Build history of the part. All positions in model axes, mm. Face numbers are marked on the shaded views. A direction names the side the tool comes from. Coordinates: 2 decimals unless noted, no trailing zeros. Write each loop counter-clockwise with the first axis right and the second up, starting at its lowest first coordinate (ties: lowest second). Pieces come first, ordered by that corner, then holes.
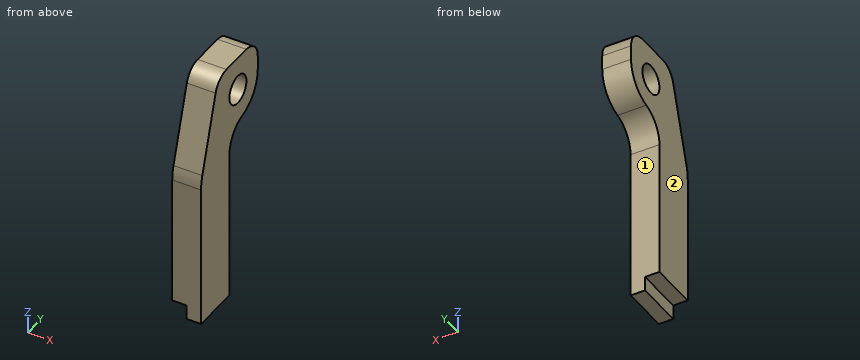
```python
from build123d import *

# Parameters (mm, degrees)
TAB_EXTRUDE_DEPTH       = 5
SKETCH2_R               = 1.5
SCREWHOLE_EXTRUDE_DEPTH = 3
STRUCTURAL_FILLETS_R    = 5


with BuildPart() as part:
    # Sketch1 → Tab extrude (new body)
    with BuildSketch(Plane(origin=(0, 116.5, 0), x_dir=(1, 0, 0), z_dir=(0, 1, 0))):
        Polygon((-4, 23.815), (-2.5, 23.815), (-2.5, 25.315), (-1, 25.315), (-1, 9.63955532), (-4, 9.63955532), align=None)
    extrude(amount=-TAB_EXTRUDE_DEPTH)

    # Sketch2 → Screwhole extrude (add)
    with BuildSketch(Plane.ZY.offset(1)):
        with BuildLine():
            Line((-9.63955532, 111.5), (-1.230909725, 114.067641584))
            ThreePointArc((-1.230909725, 114.067641584), (-0.207489417, 114.790530608), (0.185, 115.980450657))
            Line((0.185, 115.980450657), (0.185, 119.5))
            ThreePointArc((0.185, 119.5), (-0.400786438, 120.914213562), (-1.815, 121.5))
            Line((-1.815, 121.5), (-3.315, 121.5))
            ThreePointArc((-3.315, 121.5), (-5.485607855, 120.745625892), (-6.720529788, 118.807692308))
            ThreePointArc((-6.720529788, 118.807692308), (-7.779034301, 117.146606378), (-9.63955532, 116.5))
            Line((-9.63955532, 116.5), (-9.63955532, 111.5))
        make_face()
        with Locations((-3.315, 118)):
            Circle(SKETCH2_R, mode=Mode.SUBTRACT)
    extrude(amount=SCREWHOLE_EXTRUDE_DEPTH)

    # Structural fillets
    structural_fillets_edges = [part.edges().sort_by_distance(p)[0] for p in [
        (-2.5, 111.5, -9.63955532),
    ]]
    fillet(structural_fillets_edges, radius=STRUCTURAL_FILLETS_R)


solid = part.part
```
1. Flat gauge pins, fed straight in: pin 1 (1.6 mm diameter, centred on y = 114, z = -25, fed in from -X); pin 2 (1.5 mm diameter, centred on x = -3, z = -15, fed in from +Y). Where does each tip first touch, or does it go through?
Computed values:
pin 1: stops at x = -2.5
pin 2: stops at y = 116.5
2. Saw through at B-B on y = 118. List the corners of the cut face in (x, z) (3 decimals).
Computed values:
outline: (-4, -7.041) - (-1, -7.041) - (-1, -4.815) - (-4, -4.815) - close; (-4, -1.815) - (-1, -1.815) - (-1, 0.185) - (-4, 0.185) - close
3. Saw through at A-A on x = -1.8. List the corners of the cut face in (y, z) (3 decimals), plus the area to 3 significant figures.
Computed values:
outline: (111.5, -25.315) - (116.5, -25.315) - (116.5, -9.64) arc R3 cw to (118.808, -6.721) arc R3.5 ccw to (121.5, -3.315) - (121.5, -1.815) arc R2 ccw to (119.5, 0.185) - (115.98, 0.185) arc R2 ccw to (114.068, -1.231) - (111.718, -8.926) arc R5 ccw to (111.5, -10.386) - close; hole circle Ø3 at (118, -3.315)
area: 138 mm2
4. Saw through at D-D on x = -2.9. List the corners of the cut face in (y, z) (3 decimals).
Computed values:
outline: (111.5, -23.815) - (116.5, -23.815) - (116.5, -9.64) arc R3 cw to (118.808, -6.721) arc R3.5 ccw to (121.5, -3.315) - (121.5, -1.815) arc R2 ccw to (119.5, 0.185) - (115.98, 0.185) arc R2 ccw to (114.068, -1.231) - (111.718, -8.926) arc R5 ccw to (111.5, -10.386) - close; hole circle Ø3 at (118, -3.315)
5. 3-axis set-ups, long thin cutter, end or side, ignore diameter. For the marked faces 1 and 2: which of +Z, -Z, +X, -X, +Y, -Y reach the whole face in a straight line?
Computed values:
face 1: -Z, +X, -X, +Y
face 2: +Z, -Z, -X, +Y, -Y
6. Saw through at C-C on z = -20.25. List the corners of the cut face in (x, y), plus the area to 3 significant figures.
Computed values:
outline: (-4, 111.5) - (-1, 111.5) - (-1, 116.5) - (-4, 116.5) - close
area: 15.0 mm2
7. Probe line 1 along Y through (x, z) = (-2.85, -21.25); line 2 along Z through (x, y) = (-2.1, 118) (3 decimals); line 3 along Z through (x, y) = (-1.7, 117) (3 decimals). List the from-to ranges inside material, lowest first.
Computed values:
line 1: y = 111.5 to 116.5
line 2: z = -7.041 to -4.815, -1.815 to 0.185
line 3: z = -7.981 to -4.433, -2.197 to 0.185
